Verification items for the finished model (mm, model axes). Face numbers are marked on the shaded views. Round coordinates to 2 decimals unless told otherwise and drop trailing zeros. Answer as a JSON object with one key per item and string values. Group by question number.
(1) Scan lines: L1, parallel to X at y = 0.45, z = 47; L2, parallel to Z at x = -12.5, y = 1.35; L3, parallel to Z at x = -13, y = 0.5. Record each from-to range of solid material in increasing order. Write a range as from..to.
(2) Gauge pin test, flat ends, axial feed: pin 1 Ø1 at (y, z) = (5, 34.5) entering from -X; pin 2 Ø4 at (x, z) = (-3.5, 35) entering from +Y; pin 3 Ø1 at (y, z) = (3, 41.5) entering from +X; pin 4 Ø2 at (y, z) = (0.5, 44) entering from -X. Record the tip position at first contact, or that the pin passes through.
(3) Draft check along X on the marked faces 1, 2 and 3. Enter one of: released by +X, released by -X, zero draft, split by the parting line, or undercut.
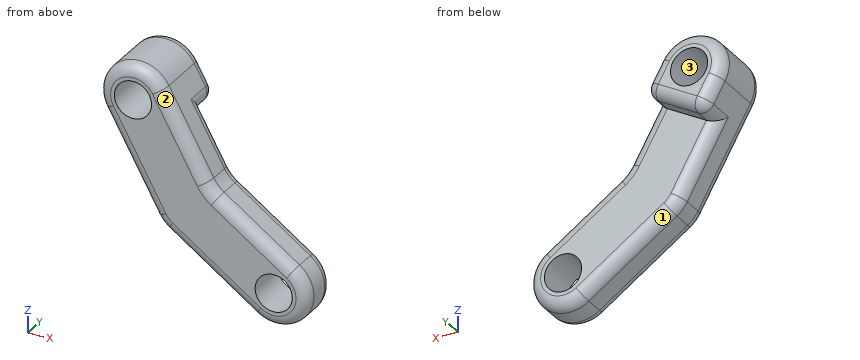
```python
from build123d import *

# Parameters (mm, degrees)
SKETCH1_R           = 1.6000000000000019
SKETCH1_R_2         = 1.6
BOSS_EXTRUDE1_DEPTH = 6
FILLET2_R           = 1
CUT_EXTRUDE1_START  = -2.3175
SKETCH3_R           = 1.6
CUT_EXTRUDE1_DEPTH  = 2.3175
FILLET3_R           = 1
FILLET4_R           = 1


with BuildPart() as part:
    # Sketch1 → Boss-Extrude1 (new body)
    with BuildSketch(Plane(origin=(0, 0, 0), x_dir=(1, 0, 0), z_dir=(0, 1, 0))):
        with BuildLine():
            Line((-14.676643190871216, 12.058848545686113), (-10.160612201428068, 3.951430072051938))
            ThreePointArc((-10.160612201428068, 3.951430072051938), (-9.770701137956143, 3.4055643719184734), (-9.26924383935776, 2.9599854477283642))
            Line((-9.26924383935776, 2.9599854477283642), (-1.6862307188325316, -2.390031581980774))
            ThreePointArc((-1.6862307188325316, -2.390031581980774), (2.3900315819807747, -1.6862307188325345), (1.6862307188325354, 2.3900315819807725))
            Line((1.6862307188325354, 2.3900315819807725), (-4.8073944342993835, 6.9714564854625545))
            ThreePointArc((-4.8073944342993835, 6.9714564854625545), (-5.308851732897766, 7.417035409652663), (-5.6987627963696905, 7.962901109786128))
            Line((-5.6987627963696905, 7.962901109786128), (-9.566013447169048, 14.90559469221669))
            ThreePointArc((-9.566013447169048, 14.90559469221669), (-13.54470139228542, 16.037536490802488), (-14.676643190871216, 12.058848545686113))
        make_face()
        with Locations(Location((-12.121328319020131, 13.482221618951401, 0), (0, 0, 270))):
            Circle(SKETCH1_R, mode=Mode.SUBTRACT)
        with Locations(Location((1.73e-15, -8.7e-16, 0), (0, 0, 270))):
            Circle(SKETCH1_R_2, mode=Mode.SUBTRACT)
    extrude(amount=BOSS_EXTRUDE1_DEPTH)

    # Fillet2
    fillet2_edges = [part.edges().sort_by_distance(p)[0] for p in [
        (-12.418627696149642, 0, -8.005139308869026),
        (-13.544701392285422, 0, -16.037536490802488),
        (-7.632388121769369, 0, -11.43424790100141),
        (-5.308851732897767, 0, -7.417035409652664),
        (-13.544701392285422, 6, -16.037536490802488),
        (-12.418627696149642, 6, -8.005139308869026),
        (-9.770701137956143, 6, -3.405564371918474),
        (-5.4777372790951455, 6, -0.28497693287379544),
        (2.390031581980775, 6, 1.686230718832534),
        (-1.5605818577334243, 6, -4.6807440337216635),
        (-5.308851732897767, 6, -7.417035409652664),
        (-1.5605818577334243, 0, -4.6807440337216635),
        (-7.632388121769369, 6, -11.43424790100141),
        (2.390031581980775, 0, 1.686230718832534),
        (-5.4777372790951455, 0, -0.28497693287379544),
        (-9.770701137956143, 0, -3.405564371918474),
    ]]
    fillet(fillet2_edges, radius=FILLET2_R)

    # Sketch3 → Cut-Extrude1 (cut)
    # profile 1 of 2: a face of its own
    with BuildSketch(Plane(origin=(0, 6, 0), x_dir=(1, 0, 0), z_dir=(0, 1, 0)).offset(CUT_EXTRUDE1_START)):
        with BuildLine():
            ThreePointArc((-5.383883568942986, 6.154351671110155), (-6.052493300407496, 6.748456903363634), (-6.572374718370062, 7.476277836874918))
            Line((-6.572374718370061, 7.476277836874918), (-8.97975555043579, 11.79813565330437))
            Line((-8.979755550435788, 11.79813565330437), (-12.343161450137215, 9.924636052596211))
            Line((-12.343161450137217, 9.92463605259621), (-9.287000279427696, 4.438053344963148))
            ThreePointArc((-9.287000279427696, 4.438053344963148), (-9.027059570446415, 4.074142878207507), (-8.692754704714162, 3.7770902620807663))
            Line((-8.692754704714162, 3.7770902620807667), (-1.1097415841889307, -1.5729267676283727))
            ThreePointArc((-1.1097415841889307, -1.5729267676283722), (1.5729267676283736, -1.1097415841889322), (1.1097415841889327, 1.5729267676283718))
            Line((1.1097415841889327, 1.5729267676283716), (-5.383883568942986, 6.154351671110155))
        make_face()
        with Locations(Location((1.73e-15, -8.7e-16, 0), (0, 0, 270))):
            Circle(SKETCH3_R, mode=Mode.SUBTRACT)
    # profile 2 of 2: a face of its own
    with BuildSketch(Plane(origin=(0, 6, 0), x_dir=(1, 0, 0), z_dir=(0, 1, 0)).offset(CUT_EXTRUDE1_START)):
        with BuildLine():
            Line((-8.97975555043579, 11.79813565330437), (-6.572374718370061, 7.476277836874918))
            ThreePointArc((-6.572374718370062, 7.476277836874918), (-6.052493300407496, 6.748456903363634), (-5.383883568942986, 6.154351671110155))
            Line((-5.383883568942986, 6.154351671110155), (1.1097415841889327, 1.5729267676283716))
            ThreePointArc((1.1097415841889327, 1.5729267676283718), (1.5729267676283736, -1.1097415841889322), (-1.1097415841889307, -1.5729267676283722))
            Line((-1.1097415841889307, -1.5729267676283727), (-8.692754704714162, 3.7770902620807667))
            ThreePointArc((-8.692754704714162, 3.7770902620807663), (-9.027059570446415, 4.074142878207507), (-9.287000279427696, 4.438053344963148))
            Line((-9.287000279427696, 4.438053344963148), (-12.343161450137217, 9.92463605259621))
            Line((-12.343161450137215, 9.924636052596211), (-13.216773372137586, 9.438012779685))
            Line((-13.216773372137586, 9.438012779685), (-10.160612201428068, 3.951430072051938))
            ThreePointArc((-10.160612201428068, 3.951430072051938), (-9.770701137956145, 3.4055643719184743), (-9.269243839357761, 2.959985447728366))
            Line((-9.269243839357761, 2.9599854477283656), (-1.6862307188325316, -2.390031581980774))
            ThreePointArc((-1.6862307188325316, -2.390031581980774), (2.3900315819807743, -1.686230718832534), (1.686230718832535, 2.390031581980772))
            Line((1.686230718832534, 2.3900315819807725), (-4.8073944342993835, 6.9714564854625545))
            ThreePointArc((-4.807394434299383, 6.971456485462554), (-5.308851732897767, 7.417035409652663), (-5.6987627963696905, 7.962901109786128))
            Line((-5.6987627963696905, 7.962901109786128), (-8.10614362843542, 12.284758926215579))
            Line((-8.10614362843542, 12.284758926215579), (-8.979755550435788, 11.79813565330437))
        make_face()
    extrude(amount=CUT_EXTRUDE1_DEPTH, mode=Mode.SUBTRACT)

    # Fillet3
    fillet3_edges = [part.edges().sort_by_distance(p)[0] for p in [
        (-6.9024532124025555, 3.6825, -10.123830018000854),
        (-5.308851732897768, 3.6825, -7.417035409652662),
        (-1.5605818577334247, 3.6825, -4.6807440337216635),
        (-5.477737279095146, 3.6825, -0.2849769328737959),
        (-11.688692786782827, 3.6825, -6.694721425868469),
        (-9.770701137956145, 3.6825, -3.405564371918474),
        (2.390031581980774, 3.6825, 1.6862307188325336),
    ]]
    fillet(fillet3_edges, radius=FILLET3_R)

    # Fillet4
    fillet4_edges = [part.edges().sort_by_distance(p)[0] for p in [
        (-12.96089836430909, 5.707106781186548, -9.580541436437505),
        (-10.661458500286502, 6, -10.86138585295029),
        (-8.362018636263915, 5.707106781186548, -12.142230269463079),
        (-13.216773372137585, 3.84125, -9.438012779685),
        (-8.106143628435422, 3.84125, -12.28475892621558),
    ]]
    fillet(fillet4_edges, radius=FILLET4_R)


with BuildPart() as body_2:
    # Mirror12: mirrored copy
    add(part.part.mirror(Plane.XY.offset(16.56331838768985)))


solid = body_2.part
```
Computed values:
{
 "1": {"L1": "-14.85..-13.67, -10.57..-9.18", "L2": "41.28..45.05, 48.16..49.51", "L3": "42.45..45.27, 47.95..49.26"},
 "2": {"pin 1": "through", "pin 2": "y = 3.68", "pin 3": "x = -5.68", "pin 4": "x = -14.53"},
 "3": {"face 1": "released by -X", "face 2": "released by +X", "face 3": "undercut"}
}
